The drawing under review shows one solid part. Ordinate dimensions are in mm from its lowest x, y, z. A direction names the side the tool comes from. Give positions to 0.01 mm unless a question says otherwise; leave off trailing zeros. Order: outer loops, then holes, each group sorted by start corner. A loop starts at its lowest first (then second) coordinate and runs counter-clockwise, first axis right, second up. Notation, with made-up numbers: (-32, -15) - (-25, -15) arc R37 ccw to (-25, 24) - close; hole circle Ø6 at (46, 84.25). An arc over 180 degrees is marked (long way). Use CSV: the item, a comma, the result in double quotes. Start each with the question number.
1. To check wall thickness, follow line 1 (Z direction, x = 89, y = 52); line 2 (Y direction, x = 50, z = 148). State the ranges of each line that lie inside material, in increasing order. Write a range as [from, to].
2. Take a section at B-B, the plane z = 120. State the section outline as (x, y) points, then the cut area to 3 significant figures.
3. Machinability: for the marked faces 1 and 2, which of the approach directions +Z, -Z, +X, -X, +Y, -Y give a long, thin tool a straight path to every point of the face, cutting with its end or side? Answer none if there is none.
4. Take a section at A-A, the plane x = 85.5. State the section outline as (y, z) points.
5. Take a section at C-C, the plane y = 115. State the section outline as (x, z) points, then the cut area to 3 significant figures.
6. For pin 1 (5 mm diameter, centred on x = 106.5, y = 93, fed in from -Z); pin 2 (12 mm diameter, centred on x = 72, z = 169.5, fed in from +Y), all flat-tipped, find the tip position at first contact; note any pin that passes through.
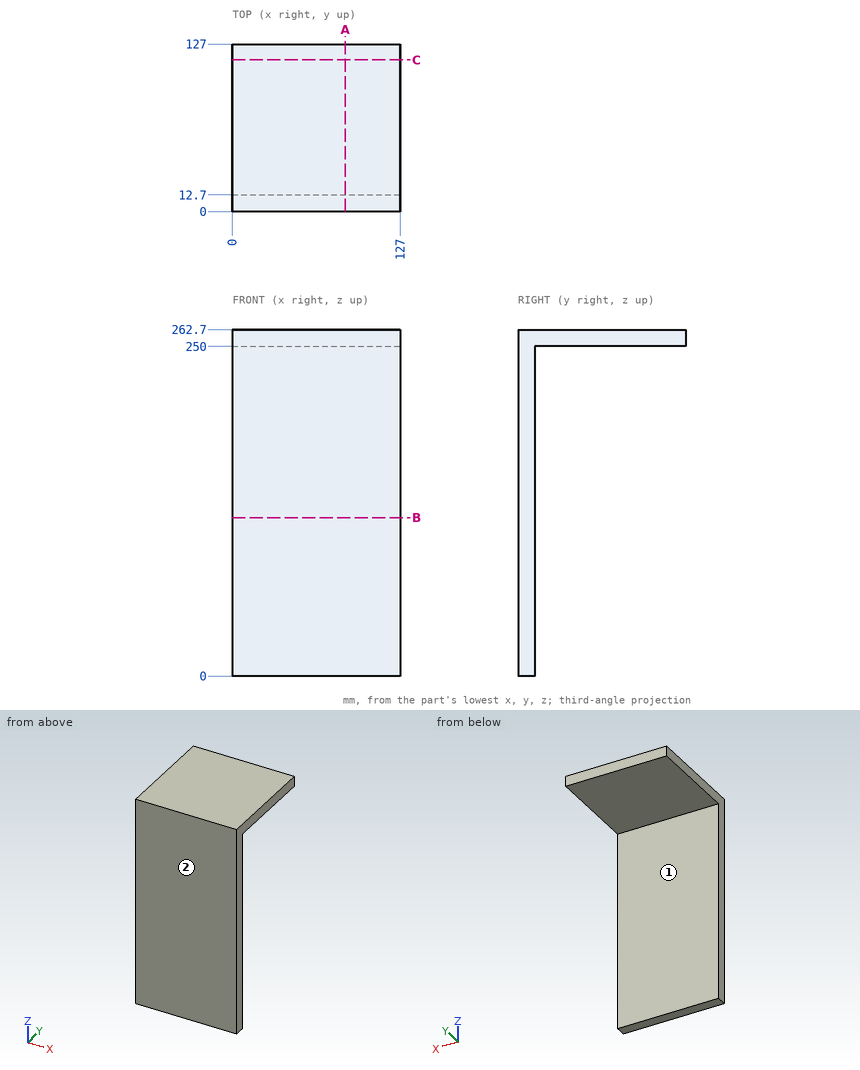
Determined:
1,line 1,"z = [250, 262.7]"
1,line 2,"y = [0, 12.7]"
2,outline,"(0, 0) - (127, 0) - (127, 12.7) - (0, 12.7) - close"
2,area,"1,610 mm²"
3,face 1,"-Z, +X, -X, +Y"
3,face 2,"+Z, -Z, +X, -X, -Y"
4,outline,"(0, 0) - (12.7, 0) - (12.7, 250) - (127, 250) - (127, 262.7) - (0, 262.7) - close"
5,outline,"(0, 250) - (127, 250) - (127, 262.7) - (0, 262.7) - close"
5,area,"1,610 mm²"
6,pin 1,"stops at z = 250"
6,pin 2,"stops at y = 12.7"
